from build123d import *

# Parameters (mm, degrees)
SKETCH5_R = 1
SKETCH4_W = 4
SKETCH4_H = 2


with BuildPart() as part:
    # Sweep1: sweep along a path in Sketch3
    with BuildLine(Plane.XY) as sweep1_path:
        Line((0, 0), (0, 90))
        Line((0, 90), (100, 90))
        Line((100, 90), (100, 0))
    # Sketch5 → Sweep1 (sweep)
    with BuildSketch(Plane(origin=(0, 0, 0), x_dir=(1, 0, 0), z_dir=(0, 1, 0))):
        Circle(SKETCH5_R)
    sweep(path=sweep1_path.line, transition=Transition.RIGHT)

    # Sketch4 → Revolve1 (revolve)
    with BuildSketch(Plane.YZ):
        with BuildLine():
            Line((0, -4.3), (0, 0))
            Line((0, 0), (-1, 0))
            Line((-1, 0), (-1, -2))
            Line((-1, -2), (-1, -5))
            Line((-1, -5), (-0.7, -5))
            ThreePointArc((-0.7, -5), (-0.205025253, -4.794974747), (0, -4.3))
        make_face()
        with Locations((-3, -1)):
            Rectangle(SKETCH4_W, SKETCH4_H)
    revolve1 = revolve(axis=Axis((0, 0, 0), (0, 1, 0)))

    # Mirror1: Revolve1 across plane
    add(revolve1.mirror(Plane(origin=(50, 0, 0), x_dir=(0, 0, 1), z_dir=(1, 0, 0))))


solid = part.part
Design review of the part built by this model. Coordinates are the model's own, in mm. A direction names the side the tool comes from. Coordinates: 2 decimals unless noted, no trailing zeros. Order: outer loops, then holes, each group sorted by start corner. A loop starts at its lowest first (then second) coordinate and runs counter-clockwise, first axis right, second up. Notation, with made-up numbers: (-35.5, 35) -> (5.5, 35) arc R25 cw to (5.5, 50) -> close; hole circle Ø5 at (11, 71.25). An arc over 180 degrees is marked (long way). One line per item, written item: value.
1) Clearance check with flat-ended pins moving along their axes: P1, Ø5, axis at y = 48.5, z = -3, coming from the +X side; P2, Ø4.5, axis at x = 101, z = -0.5, coming from the +Y side. State where each tip first meets the part, or that it passes through.
Output values:
P1: stops at x = 100.87
P2: stops at y = 91
2) We need section A-A, the plane y = 63. Give the boundary of the cut face in (x, z).
Output values:
outline: circle Ø2 at (0, 0); circle Ø2 at (100, 0)
3) To check wall thickness, follow probe 1 along X at (y, z) = (17, -0.5); probe 2 along Y at (x, z) = (96, 2); probe 3 along Y at (x, z) = (101, 0.5). State the ranges of each line that lie inside material, in increasing order. Write a range as [from, to].
Output values:
probe 1: x = [-0.87, 0.87], [99.13, 100.87]
probe 2: y = [-1, -0.02]
probe 3: y = [-5, 0]
4) Machinability: for faces 1 (the face through (2, -3, 0)), 2 (the face through (100, -5, 0)), which of the approach directions +Z, -Z, +X, -X, +Y, -Y give a long, thin tool a straight path to every point of the face, cutting with its end or side? Answer none if there is none.
Output values:
face 1: -Y
face 2: +Z, -Z, +X, -X, -Y
5) We need section B-B, the plane x = 10.5. Give the boundary of the cut face in (y, z).
Output values:
outline: circle Ø2 at (90, 0)
